For this review, take the finished solid that the model builds, in its own axes (mm). A direction names the side the tool comes from. Round coordinates to 2 decimals unless told otherwise and drop trailing zeros. Order: outer loops, then holes, each group sorted by start corner. A loop starts at its lowest first (then second) coordinate and runs counter-clockwise, first axis right, second up. Notation, with made-up numbers: (-26.5, 54.25) -> (8.5, 54.25) arc R32 cw to (8.5, 82.25) -> close; hole circle Ø4 at (-27.5, 71.5). An arc over 180 degrees is marked (long way). Answer in a Markdown table with one row per item.
```python
from build123d import *

# Parameters (mm, degrees)
F1_ANGLE    = 180
F2_T4_ANGLE = 243.6352501502
F2_S5_R     = 11.8
F2_T6_DEPTH = 16
F3_T4_ANGLE = 243.2500896942
F3_S5_R     = 11.8
F3_T6_DEPTH = 16
F4_T4_ANGLE = 243.7164036037
F4_S5_R     = 11.8
F4_T6_DEPTH = 16
F5_T4_ANGLE = 243.7164036037
F5_S5_R     = 11.8
F5_T6_DEPTH = 16
F6_T4_ANGLE = 310.0876573575
F6_S5_R     = 6.8
F6_T6_DEPTH = 11


# Not quite as in the source:
# - a fillet or chamfer that OpenCascade refuses, or shapes differently, is made with other operations: its cross-section is extruded or revolved along the edge and cut away or added


with BuildPart() as f1:
    # F0 (on Top) → F1 (revolve)
    with BuildSketch(Plane.XY):
        Polygon((-11.8, 5.65), (-11.8, 6.65), (-13.8, 6.65), (-13.8, 0), (-7.8, -10.95), (-6.8, -10.95), (-6.8, -9.45), (-4.8, -9.45), (-4.8, -7.45), (-9.8, 1), (-11.8, 1), (-11.8, 2), (-9.8, 2), (-9.8, 5.65), align=None)
        Polygon((-13.8, 6.65), (-11.8, 6.65), (-9.8, 6.65), (-9.8, 8.65), (-13.8, 8.65), align=None)
    revolve(axis=Axis((0, 0, 0), (0, -1, 0)), revolution_arc=F1_ANGLE)

    # F2: chamfer of 2.1 on 1 edges, made by hand


with BuildPart() as f2_tool2:
    # F2_s3 → F2_t4 (revolve)
    with BuildSketch(Plane(origin=(0, 0, 0), x_dir=(0, 1, 0), z_dir=(0.5272172108, 0, 0.849730553))):
        Polygon((-0.8073066866, 8.7305877594), (1, 11.9), (1, 9.8), align=None)
    revolve(axis=Axis((0, 1, 0), (0, -1, 0)), revolution_arc=F2_T4_ANGLE)

    # F2_s5 → F2_t6 (intersect, symmetric)
    with BuildSketch(Plane.XZ.offset(-0.1)):
        Circle(F2_S5_R)
    extrude(amount=F2_T6_DEPTH, both=True, mode=Mode.INTERSECT)


with BuildPart() as f1_1:
    add(f1.part)

    # F2_t1: cut F2_tool2
    add(f2_tool2.part, mode=Mode.SUBTRACT)

    # F3: chamfer of 2.1 on 1 edges, made by hand


with BuildPart() as f3_tool2:
    # F3_s3 → F3_t4 (revolve)
    with BuildSketch(Plane(origin=(0, 0, 0), x_dir=(0, 1, 0), z_dir=(0.5243581586, 0, 0.8514978107))):
        Polygon((5.65, 11.9), (3.55, 9.8), (5.65, 9.8), align=None)
    revolve(axis=Axis((0, 5.65, 0), (0, -1, 0)), revolution_arc=F3_T4_ANGLE)

    # F3_s5 → F3_t6 (intersect, symmetric)
    with BuildSketch(Plane.XZ.offset(-4.6)):
        Circle(F3_S5_R)
    extrude(amount=F3_T6_DEPTH, both=True, mode=Mode.INTERSECT)


with BuildPart() as f1_2:
    add(f1_1.part)

    # F3_t1: cut F3_tool2
    add(f3_tool2.part, mode=Mode.SUBTRACT)

    # F4: chamfer of 2.1 x 1 on 1 edges, made by hand


with BuildPart() as f4_tool2:
    # F4_s3 → F4_t4 (revolve)
    with BuildSketch(Plane(origin=(0, 0, 0), x_dir=(0, 1, 0), z_dir=(0.5278188556, 0, 0.849356966))):
        Polygon((7.65, 9.8), (6.65, 11.9), (6.65, 9.8), align=None)
    revolve(axis=Axis((0, 6.65, 0), (0, -1, 0)), revolution_arc=F4_T4_ANGLE)

    # F4_s5 → F4_t6 (intersect, symmetric)
    with BuildSketch(Plane.XZ.offset(-7.2)):
        Circle(F4_S5_R)
    extrude(amount=F4_T6_DEPTH, both=True, mode=Mode.INTERSECT)


with BuildPart() as f1_3:
    add(f1_2.part)

    # F4_t1: cut F4_tool2
    add(f4_tool2.part, mode=Mode.SUBTRACT)

    # F5: chamfer of 2.1 x 1 on 1 edges, made by hand


with BuildPart() as f5_tool2:
    # F5_s3 → F5_t4 (revolve)
    with BuildSketch(Plane(origin=(0, 0, 0), x_dir=(0, 1, 0), z_dir=(0.5278188556, 0, 0.849356966))):
        Polygon((3, 9.8), (2, 11.9), (2, 9.8), align=None)
    revolve(axis=Axis((0, 2, 0), (0, -1, 0)), revolution_arc=F5_T4_ANGLE)

    # F5_s5 → F5_t6 (intersect, symmetric)
    with BuildSketch(Plane.XZ.offset(-2.5)):
        Circle(F5_S5_R)
    extrude(amount=F5_T6_DEPTH, both=True, mode=Mode.INTERSECT)


with BuildPart() as f1_4:
    add(f1_3.part)

    # F5_t1: cut F5_tool2
    add(f5_tool2.part, mode=Mode.SUBTRACT)

    # F6: chamfer of 2.1 x 1 on 1 edges, made by hand


with BuildPart() as f6_tool2:
    # F6_s3 → F6_t4 (revolve)
    with BuildSketch(Plane(origin=(0, 0, 0), x_dir=(0, 1, 0), z_dir=(0.9066308057, 0, 0.4219248537))):
        Polygon((-8.45, 4.8), (-9.45, 6.9), (-9.45, 4.8), align=None)
    revolve(axis=Axis((0, -9.45, 0), (0, -1, 0)), revolution_arc=F6_T4_ANGLE)

    # F6_s5 → F6_t6 (intersect, symmetric)
    with BuildSketch(Plane.XZ.offset(8.9)):
        Circle(F6_S5_R)
    extrude(amount=F6_T6_DEPTH, both=True, mode=Mode.INTERSECT)


with BuildPart() as f1_5:
    add(f1_4.part)

    # F6_t1: cut F6_tool2
    add(f6_tool2.part, mode=Mode.SUBTRACT)


solid = f1_5.part
```
Q1. Take a section at D-D, the plane y = 4.5. Write out the cut boundary in (x, z).
Answer key:
| item | result |
|---|---|
| outline | (-13.8, 0) arc R13.8 ccw to (13.8, 0) -> (10.75, 0) arc R10.75 cw to (-10.75, 0) -> close |
Q2. To check wall thickness, follow probe 1 along X at (y, z) = (-2.25, -6.5); probe 2 along Y at (x, z) = (11.25, -3); probe 3 along Y at (x, z) = (-5.75, -8.25). State the ranges of each line that lie inside material, in increasing order.
Answer key:
| item | result |
|---|---|
| probe 1 | x = -10.76 to -4.45, 4.45 to 10.76 |
| probe 2 | y = -3.94 to 0.85, 2.12 to 5.39, 6.77 to 8.65 |
| probe 3 | y = -6.83 to -0.05, 2.88 to 3.81, 7.53 to 8.65 |
Q3. The part is to be moulded in two halves that separate along Y. For faces 1 (the face through (10, -1, 0)), 2 (the face through (-0.223, 7.485, -10.145)), 3 (the face through (-0.2, -0.7, -8.92)), 4 (the face through (-0.22, -6.77, -10.09)), say which applies: +Y half, -Y half, draft (parallel to the pull), parting line (faces both ways), or undercut.
Answer key:
| item | result |
|---|---|
| face 1 | draft |
| face 2 | undercut |
| face 3 | undercut |
| face 4 | -Y half |
Q4. Clearance check with flat-ended pins moving along their axes: pin 1 Ø1 at (x, y) = (-8.5, -8) entering from -Z; pin 2 Ø1.5 at (y, z) = (1.5, -5) entering from -X; pin 3 Ø10 at (x, y) = (-8, -3.5) entering from -Z. State where each tip first meets the part, or that it passes through.
Answer key:
| item | result |
|---|---|
| pin 1 | stops at z = -5.12 |
| pin 2 | stops at x = -13.13 |
| pin 3 | stops at z = -13.07 |
Q5. Tool access review of faces 5 (the face through (-0.215, 8.157, -9.798)), 6 (the face through (-0.259, 1.488, -11.797)), 7 (the face through (-0.1, -10.2, -6.8)): name each direction out of +Z, -Z, +X, -X, +Y, -Y from which nothing blocks a thin tool from reaching the whole face with its end or side.
Answer key:
| item | result |
|---|---|
| face 5 | +Z, +Y |
| face 6 | +Z |
| face 7 | +Z, -Y |
Q6. Take a section at A-A, the plane x = 0. Write out the cut boundary in (y, z), then the cut area to 3 significant figures.
Answer key:
| item | result |
|---|---|
| outline | (-10.95, -7.8) -> (0, -13.8) -> (8.65, -13.8) -> (8.65, -9.8) -> (7.65, -9.8) -> (6.7, -11.8) -> (5.55, -11.8) -> (3.55, -9.8) -> (3, -9.8) -> (2.05, -11.8) -> (0.94, -11.8) -> (-0.81, -8.73) -> (-7.45, -4.8) -> (-8.45, -4.8) -> (-9.4, -6.8) -> (-10.95, -6.8) -> close |
| area | 69.9 mm^2 |
Q7. Take a section at C-C, the plane z = -11.5. Give the number of separate pieces and of enclosed holes in the cut face, then the cut area to 3 significant figures.
Answer key:
| item | result |
|---|---|
| separate pieces | 1 |
| enclosed holes | 2 |
| area | 159 mm^2 |
Q8. Take a section at B-B, the plane y = 1.75. Write out the cut boundary in (x, z), then the cut area to 3 significant figures.
Answer key:
| item | result |
|---|---|
| outline | (-13.8, 0) arc R13.8 ccw to (13.8, 0) -> (11.8, 0) arc R11.8 cw to (-11.8, 0) -> close |
| area | 80.4 mm^2 |
